```python
from build123d import *

# Parameters (mm, degrees)
SKETCH1_W               = 25.4
SKETCH1_H               = 25.4
BOSS_EXTRUDE1_DEPTH     = 3.175
SKETCH2_W               = 3.175
SKETCH2_H               = 25.4
BOSS_EXTRUDE2_DEPTH     = 22.225
F_1_4_CLEARANCE_HOLE2_D = 6.7564
F_1_4_CLEARANCE_HOLE1_D = 6.7564


with BuildPart() as part:
    # Sketch1 → Boss-Extrude1 (new body)
    with BuildSketch(Plane(origin=(0, 0, 0), x_dir=(1, 0, 0), z_dir=(0, 1, 0))):
        Rectangle(SKETCH1_W, SKETCH1_H)
    extrude(amount=BOSS_EXTRUDE1_DEPTH)

    # Sketch2 → Boss-Extrude2 (add)
    with BuildSketch(Plane(origin=(0, 3.175, 0), x_dir=(1, 0, 0), z_dir=(0, 1, 0))):
        with Locations((-11.1125, 0)):
            Rectangle(SKETCH2_W, SKETCH2_H)
        with Locations((11.1125, 0)):
            Rectangle(SKETCH2_W, SKETCH2_H)
    extrude(amount=BOSS_EXTRUDE2_DEPTH)

    # 1/4 Clearance Hole2 (through all)
    with Locations(Plane(origin=(0, 3.175, 0), x_dir=(1, 0, 0), z_dir=(0, 1, 0))):
        with Locations((1.905, 5.08), (-1.905, -5.08)):
            Hole(F_1_4_CLEARANCE_HOLE2_D / 2)

    # 1/4 Clearance Hole1 (through all)
    with Locations(Plane.ZY.offset(12.7)):
        with Locations((-3.175, 12.7)):
            Hole(F_1_4_CLEARANCE_HOLE1_D / 2)


solid = part.part
```
CAD build for the part. Positions are in the model's coordinates, mm. A direction names the side the tool comes from. Round coordinates to 2 decimals unless told otherwise and drop trailing zeros. Write each loop counter-clockwise with the first axis right and the second up, starting at its lowest first coordinate (ties: lowest second). Pieces come first, ordered by that corner, then holes. Notation, with made-up numbers: (-39.75, -5.75) -> (-29.75, -5.75) arc R22 ccw to (-29.75, 0.25) -> close; hole circle Ø11 at (7, -2.5). An arc over 180 degrees is marked (long way). Answer in a Markdown table with one row per item. Add a question column.
Item 1: Mould opens along Z. For faces 1 (the face through (11.13, 9.7, -4.73)), 2 (the face through (-1, 2, 12.7)), 3 (the face through (11, 25.4, 0)) say: pulls with the +Z half, pulls with the -Z half, needs draft (parallel to the pull), parting line crosses it, or undercut.
Item 2: Saw through at A-A, the plane y = 12.7. Write the cut outline in (x, z) (3 decimals), then the cut area to 3 significant figures.
Item 3: Drop a flat-ended pin along its axis: pin 1 Ø8 at (x, z) = (-1.905, 5.08) entering from +Y (3 decimals). Give the stop position or say it passes through.
Item 4: Drill centre lines: line 1 (X direction, y = 24.25, z = 7.75) (3 decimals); line 2 (X direction, y = 1.75, z = 5); line 3 (Y direction, x = 4.25, z = -10.25) (3 decimals). Where is each one in solid material? Low to high. Write a range as from..to.
Item 5: Saw through at C-C, the plane x = 3.75. Write the cut outline in (y, z) (3 decimals).
Item 6: Saw through at D-D, the plane y = 18. Write the cut outline in (x, z) (3 decimals).
Item 7: Which spindle directions (+Z, -Z, +X, -X, +Y, -Y) get a long thin tool onto all of the face, cutting with end or side? Do faces 4 (the face through (0, 3.175, 0)), 5 (the face through (12.7, 13, 3)). Say none if no direction does.
Item 8: Saw through at B-B, the plane z = 5.08. Write the cut outline in (x, y) (3 decimals), then the cut area to 3 significant figures.
Findings below:
| question | item | result |
|---|---|---|
| 1 | face 1 | undercut |
| 1 | face 2 | pulls with the +Z half |
| 1 | face 3 | needs draft |
| 2 | outline | (-12.7, -12.7) -> (-9.525, -12.7) -> (-9.525, -6.553) -> (-12.7, -6.553) -> close; (-12.7, 0.203) -> (-9.525, 0.203) -> (-9.525, 12.7) -> (-12.7, 12.7) -> close; (9.525, -12.7) -> (12.7, -12.7) -> (12.7, -6.553) -> (9.525, -6.553) -> close; (9.525, 0.203) -> (12.7, 0.203) -> (12.7, 12.7) -> (9.525, 12.7) -> close |
| 2 | area | 118 mm^2 |
| 3 | pin 1 | stops at y = 3.175 |
| 4 | line 1 | x = -12.7..-9.525, 9.525..12.7 |
| 4 | line 2 | x = -12.7..-5.28, 1.47..12.7 |
| 4 | line 3 | y = 0..3.175 |
| 5 | outline | (0, -12.7) -> (3.175, -12.7) -> (3.175, -7.91) -> (0, -7.91) -> close; (0, -2.25) -> (3.175, -2.25) -> (3.175, 12.7) -> (0, 12.7) -> close |
| 6 | outline | (-12.7, -12.7) -> (-9.525, -12.7) -> (-9.525, 12.7) -> (-12.7, 12.7) -> close; (9.525, -12.7) -> (12.7, -12.7) -> (12.7, 12.7) -> (9.525, 12.7) -> close |
| 7 | face 4 | +Z, -Z, +Y |
| 7 | face 5 | +Z, -Z, +X, +Y, -Y |
| 8 | outline | (-12.7, 0) -> (-5.283, 0) -> (-5.283, 3.175) -> (-9.525, 3.175) -> (-9.525, 25.4) -> (-12.7, 25.4) -> close; (1.473, 0) -> (12.7, 0) -> (12.7, 25.4) -> (9.525, 25.4) -> (9.525, 3.175) -> (1.473, 3.175) -> close |
| 8 | area | 200 mm^2 |
